Model file for the job. Use its own axes, mm. Coordinates: 2 decimals unless noted, no trailing zeros. Order: outer loops, then holes, each group sorted by start corner. A loop starts at its lowest first (then second) coordinate and runs counter-clockwise, first axis right, second up. Notation, with made-up numbers: (72.25, 69.5) -> (79.25, 69.5) arc R18 ccw to (79.25, 98.5) -> close; hole circle Ø6 at (-17.5, 82). An arc over 180 degrees is marked (long way). Return JSON: item names as keys, results as strings. Group by question number.
1) Flat gauge pins, fed straight in: pin 1 (1.1 mm diameter, centred on x = 5.5, z = 2, fed in from +Y); pin 2 (0.9 mm diameter, centred on y = 171.5, z = 2, fed in from +X); pin 3 (0.5 mm diameter, centred on x = 5.5, z = 2, fed in from -Y). Where does each tip first touch, or does it go through?
2) Cut at B-B (y = 153). Write the cut outline in (x, z).
3) Cut at A-A (x = 53.5). Write the cut outline in (y, z).
4) Probe line 1 (X direction, y = 103.5, z = 0.8); line 2 (Y direction, x = 81.5, z = 2.3); line 3 (Y direction, x = 68.5, z = 2.3). List the from-to ranges inside material, lowest first.
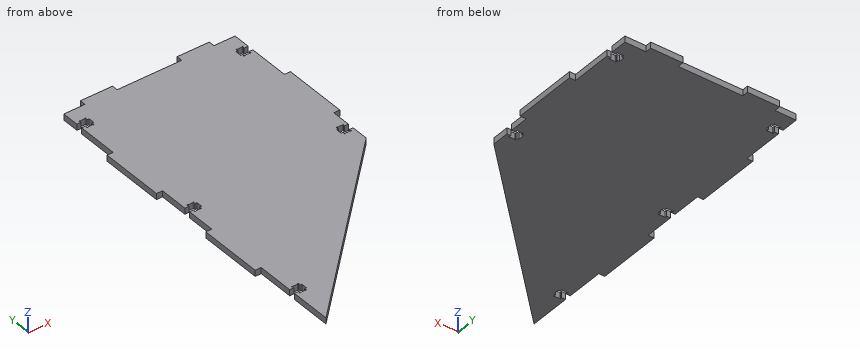
from build123d import *

# Parameters (mm, degrees)
CROQUIS1_W              = 16
CROQUIS1_H              = 3
SALIENTE_EXTRUIR1_DEPTH = 3
CORTAR_EXTRUIR1_DEPTH   = 195.118520497


with BuildPart() as part:
    # Croquis1 → Saliente-Extruir1 (new body)
    with BuildSketch(Plane.XY):
        Polygon((85, 106), (85, 85), (0, 0), (0, 42), (-3, 42), (-3, 74), (0, 74), (0, 106), (-3, 106), (-3, 138), (0, 138), (0, 170), (85, 170), (85, 138), (88, 138), (88, 106), align=None)
        with Locations((66.5, 171.5)):
            Rectangle(CROQUIS1_W, CROQUIS1_H)
        with Locations((18.5, 171.5)):
            Rectangle(CROQUIS1_W, CROQUIS1_H)
    extrude(amount=SALIENTE_EXTRUIR1_DEPTH)

    # Croquis2 → Cortar-Extruir1 (cut, through all)
    with BuildSketch(Plane.XY.offset(3)):
        with BuildLine():
            Line((2, 91.5), (0, 91.5))
            Line((0, 91.5), (0, 88.5))
            Line((0, 88.5), (2, 88.5))
            Line((2, 88.5), (2, 87.75))
            ThreePointArc((2, 87.75), (1.823223305, 87.323223305), (2.25, 87.5))
            Line((2.25, 87.5), (4.75, 87.5))
            ThreePointArc((4.75, 87.5), (5.176776695, 87.323223305), (5, 87.75))
            Line((5, 87.75), (5, 88.5))
            Line((5, 88.5), (6, 88.5))
            Line((6, 88.5), (6, 91.5))
            Line((6, 91.5), (5, 91.5))
            Line((5, 91.5), (5, 92.25))
            ThreePointArc((5, 92.25), (5.176776695, 92.676776695), (4.75, 92.5))
            Line((4.75, 92.5), (2.25, 92.5))
            ThreePointArc((2.25, 92.5), (1.823223305, 92.676776695), (2, 92.25))
            Line((2, 92.25), (2, 91.5))
        make_face()
        with BuildLine():
            Line((2, 161.5), (0, 161.5))
            Line((0, 161.5), (0, 158.5))
            Line((0, 158.5), (2, 158.5))
            Line((2, 158.5), (2, 157.75))
            ThreePointArc((2, 157.75), (1.823223305, 157.323223305), (2.25, 157.5))
            Line((2.25, 157.5), (4.75, 157.5))
            ThreePointArc((4.75, 157.5), (5.176776695, 157.323223305), (5, 157.75))
            Line((5, 157.75), (5, 158.5))
            Line((5, 158.5), (6, 158.5))
            Line((6, 158.5), (6, 161.5))
            Line((6, 161.5), (5, 161.5))
            Line((5, 161.5), (5, 162.25))
            ThreePointArc((5, 162.25), (5.176776695, 162.676776695), (4.75, 162.5))
            Line((4.75, 162.5), (2.25, 162.5))
            ThreePointArc((2.25, 162.5), (1.823223305, 162.676776695), (2, 162.25))
            Line((2, 162.25), (2, 161.5))
        make_face()
        with BuildLine():
            Line((83, 158.5), (85, 158.5))
            Line((85, 158.5), (85, 161.5))
            Line((85, 161.5), (83, 161.5))
            Line((83, 161.5), (83, 162.25))
            ThreePointArc((83, 162.25), (83.176776695, 162.676776695), (82.75, 162.5))
            Line((82.75, 162.5), (80.25, 162.5))
            ThreePointArc((80.25, 162.5), (79.823223305, 162.676776695), (80, 162.25))
            Line((80, 162.25), (80, 161.5))
            Line((80, 161.5), (79, 161.5))
            Line((79, 161.5), (79, 158.5))
            Line((79, 158.5), (80, 158.5))
            Line((80, 158.5), (80, 157.75))
            ThreePointArc((80, 157.75), (79.823223305, 157.323223305), (80.25, 157.5))
            Line((80.25, 157.5), (82.75, 157.5))
            ThreePointArc((82.75, 157.5), (83.176776695, 157.323223305), (83, 157.75))
            Line((83, 157.75), (83, 158.5))
        make_face()
        with BuildLine():
            Line((2, 23.5), (0, 23.5))
            Line((0, 23.5), (0, 20.5))
            Line((0, 20.5), (2, 20.5))
            Line((2, 20.5), (2, 19.75))
            ThreePointArc((2, 19.75), (1.823223305, 19.323223305), (2.25, 19.5))
            Line((2.25, 19.5), (4.75, 19.5))
            ThreePointArc((4.75, 19.5), (5.176776695, 19.323223305), (5, 19.75))
            Line((5, 19.75), (5, 20.5))
            Line((5, 20.5), (6, 20.5))
            Line((6, 20.5), (6, 23.5))
            Line((6, 23.5), (5, 23.5))
            Line((5, 23.5), (5, 24.25))
            ThreePointArc((5, 24.25), (5.176776695, 24.676776695), (4.75, 24.5))
            Line((4.75, 24.5), (2.25, 24.5))
            ThreePointArc((2.25, 24.5), (1.823223305, 24.676776695), (2, 24.25))
            Line((2, 24.25), (2, 23.5))
        make_face()
        with BuildLine():
            Line((83.099943711, 93.5), (85, 93.5))
            Line((85, 93.5), (85, 96.5))
            Line((85, 96.5), (83.099943711, 96.5))
            Line((83.099943711, 96.5), (83.099943711, 97.25))
            ThreePointArc((83.099943711, 97.25), (83.276720406, 97.676776695), (82.849943711, 97.5))
            Line((82.849943711, 97.5), (80.349943711, 97.5))
            ThreePointArc((80.349943711, 97.5), (79.923167016, 97.676776695), (80.099943711, 97.25))
            Line((80.099943711, 97.25), (80.099943711, 96.5))
            Line((80.099943711, 96.5), (79.099943711, 96.5))
            Line((79.099943711, 96.5), (79.099943711, 93.5))
            Line((79.099943711, 93.5), (80.099943711, 93.5))
            Line((80.099943711, 93.5), (80.099943711, 92.75))
            ThreePointArc((80.099943711, 92.75), (79.923167016, 92.323223305), (80.349943711, 92.5))
            Line((80.349943711, 92.5), (82.849943711, 92.5))
            ThreePointArc((82.849943711, 92.5), (83.276720406, 92.323223305), (83.099943711, 92.75))
            Line((83.099943711, 92.75), (83.099943711, 93.5))
        make_face()
    extrude(amount=-CORTAR_EXTRUIR1_DEPTH, mode=Mode.SUBTRACT)


solid = part.part
Answers below:
{
 "1": {"pin 1": "stops at y = 170", "pin 2": "stops at x = 74.5", "pin 3": "stops at y = 5.25"},
 "2": {"outline": "(0, 0) -> (85, 0) -> (85, 3) -> (0, 3) -> close"},
 "3": {"outline": "(53.5, 0) -> (170, 0) -> (170, 3) -> (53.5, 3) -> close"},
 "4": {"line 1": "x = 0 to 85", "line 2": "y = 81.5 to 92.5, 97.5 to 157.5, 162.5 to 170", "line 3": "y = 68.5 to 173"}
}
